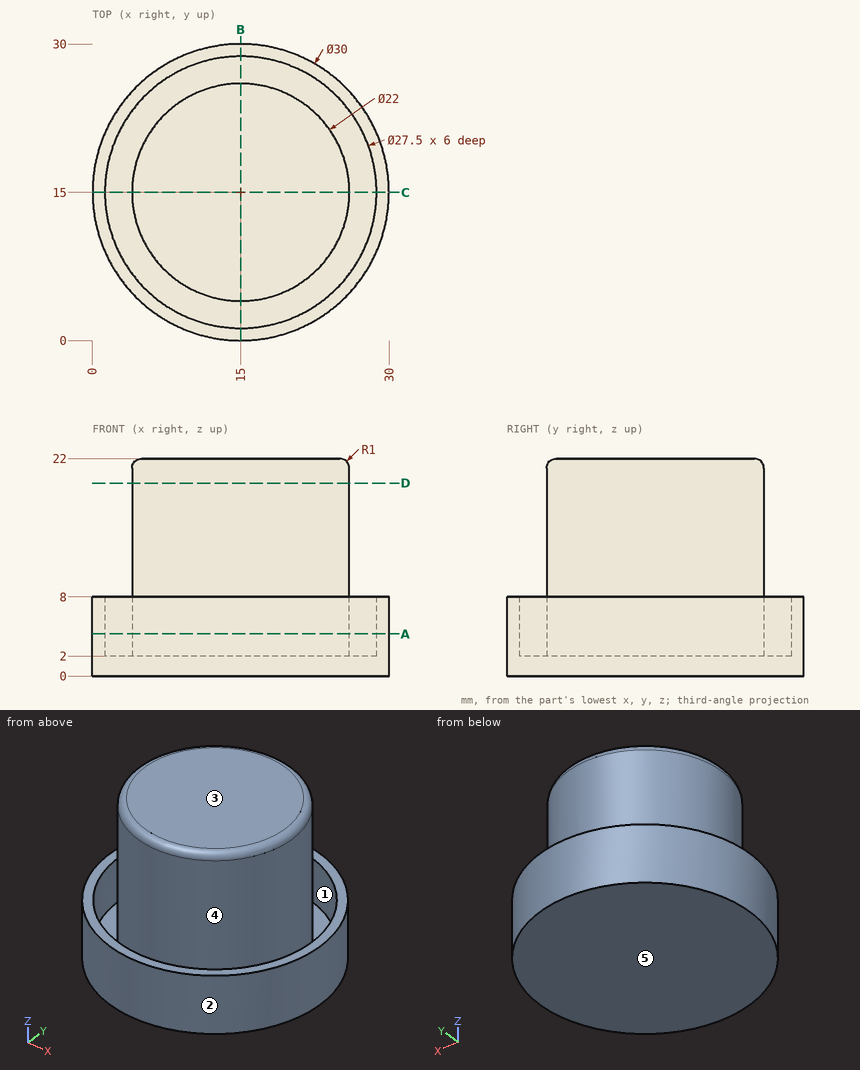
Here's the drawing with two shaded views (mm, measured from the low corner). I have some questions. A direction names the side the tool comes from. Round coordinates to 2 decimals unless told otherwise and drop trailing zeros. Write each loop counter-clockwise with the first axis right and the second up, starting at its lowest first coordinate (ties: lowest second). Pieces come first, ordered by that corner, then holes. Notation, with made-up numbers: M -17,-27 L 34,-27 A29 ccw 34,-7 Z; hole C -9,46.25 d3. An arc over 180 degrees is marked long. Use CSV: the item, a comma, the result in double quotes.
(1) Imagine slicing it at B-B (x = 15). Write out the boundary of the cut face in (y, z).
Check values:
outline,"M 0,0 L 30,0 L 30,8 L 28.75,8 L 28.75,2 L 26,2 L 26,21 A1 ccw 25,22 L 5,22 A1 ccw 4,21 L 4,2 L 1.25,2 L 1.25,8 L 0,8 Z"
(2) I'm going to push flat-ended pins straight in: pin 1 (8 mm diameter, centred on x = 9.5, z = 11, fed in from -Y); pin 2 (6 mm diameter, centred on y = 10, z = 10, fed in from -X); pin 3 (12 mm diameter, centred on x = 5, z = 19.5, fed in from +Y). Where does each tip first touch, or does it pass through?
Check values:
pin 1,"y = 0.27"
pin 2,"x = 0.26"
pin 3,"y = 25.25"
(3) On a 3-axis mill with a long thin cutter (end or side, diameter ignored), from which of +Z, -Z, +X, -X, +Y, -Y can I reach the whole of each face in a straight line? I mean the marked faces 4 and 5. Say none if no direction works.
Check values:
face 4,"+Z"
face 5,"-Z, +X, -X, +Y, -Y"
(4) Imagine slicing it at D-D (z = 19.5). Write out the boundary of the cut face in (x, y).
Check values:
outline,"C 15,15 d22"
(5) Imagine slicing it at A-A (z = 4.25). Write out the boundary of the cut face in (x, y).
Check values:
outline,"C 15,15 d30; C 15,15 d22; hole C 15,15 d27.5"
(6) I need wall thicknesses on line 1 along Y through (x, z) = (15, 4.55); line 2 along X through (y, z) = (22, 2.5); line 3 along Y through (x, z) = (17, 2.5). Which ranges of each line are inside material? Lowest first, please.
Check values:
line 1,"0 to 1.25, 4 to 26, 28.75 to 30"
line 2,"1.73 to 3.17, 6.51 to 23.49, 26.83 to 28.27"
line 3,"0.13 to 1.4, 4.18 to 25.82, 28.6 to 29.87"
(7) We'd pull the mould along X, two halves only. Please class the marked faces 1, 2 and 3: +X half, -X half, draft (parallel to the pull), parting line (faces both ways), or undercut.
Check values:
face 1,"undercut"
face 2,"parting line"
face 3,"draft"
